from build123d import *

# Parameters (mm, degrees)
SKETCH012_W             = 34.7
SKETCH012_H             = 9.5
PAD002_DEPTH            = 10.2
SKETCH013_W             = 34.7
SKETCH013_H             = 8
POCKET010_DEPTH         = 8.4
SKETCH014_W             = 11.3
SKETCH014_H             = 8
PAD003_DEPTH            = 3.8
SKETCH015_R             = 1.5
PAD004_DEPTH            = 7.5
FILLET002_R             = 0.5
SKETCH016_W             = 8.8
SKETCH016_H             = 6.75
POCKET011_DEPTH         = 3.81
SKETCH018_W             = 1.25
SKETCH018_H             = 4
POCKET012_DEPTH         = 1.25
PAD005_DEPTH            = 2.56
SKETCH019_R             = 1.9
PAD006_DEPTH            = 5
SKETCH020_R             = 1.05
POCKET014_DEPTH         = 2.56
SKETCH021_R             = 0.75
POCKET015_DEPTH         = 5
SKETCH022_W             = 1
SKETCH022_H             = 9.5
POCKET016_DEPTH         = 0.3
SKETCH023_W             = 1
SKETCH023_H             = 10.2
POCKET017_DEPTH         = 0.3
FILLET003_R             = 0.2
FILLET004_R             = 0.2
SKETCH036_R             = 1.625
PAD012_DEPTH            = 4
FILLET008_R             = 0.5
FILLET020_R             = 0.5
PAD161_DEPTH            = 1
BODY002_ROLL_ANGLE      = -90
BODY002_PLACEMENT_ANGLE = -90


with BuildPart() as part:
    # Sketch012 → Pad002 (new body)
    with BuildSketch(Plane.XY):
        with Locations((-17.35, 0)):
            Rectangle(SKETCH012_W, SKETCH012_H)
    extrude(amount=PAD002_DEPTH)

    # Sketch013 (on Face6 of Pad002) → Pocket010 (cut)
    with BuildSketch(Plane.XY.offset(10.2)):
        with Locations((-17.35, 0.75)):
            Rectangle(SKETCH013_W, SKETCH013_H)
    extrude(amount=-POCKET010_DEPTH, mode=Mode.SUBTRACT)

    # Sketch014 (on Face6 of Pocket010) → Pad003 (join)
    with BuildSketch(Plane.XY.offset(1.8)):
        with Locations((-12.75, 0.75)):
            Rectangle(SKETCH014_W, SKETCH014_H)
    extrude(amount=PAD003_DEPTH)

    # Sketch015 (on Face6 of Pad003) → Pad004 (join)
    with BuildSketch(Plane.XY.offset(1.8)):
        with Locations((-22, 0.75)):
            Circle(SKETCH015_R)
    extrude(amount=PAD004_DEPTH)

    # Fillet002
    fillet002_edges = [part.edges().sort_by_distance(p)[0] for p in [
        (-17.35, -4.75, 0),
        (-34.7, -4.75, 5.1),
        (-34.7, 0, 0),
        (0, -4.75, 5.1),
        (0, 0, 0),
    ]]
    fillet(fillet002_edges, radius=FILLET002_R)

    # Sketch016 (on Face14 of Fillet002) → Pocket011 (cut)
    with BuildSketch(Plane.XY.offset(5.6)):
        with Locations((-12.75, 0.125)):
            Rectangle(SKETCH016_W, SKETCH016_H)
    extrude(amount=-POCKET011_DEPTH, mode=Mode.SUBTRACT)

    # Sketch018 (on Face13 of Pocket011) → Pocket012 (cut)
    with BuildSketch(Plane.XY.offset(5.6)):
        with Locations((-7.725, 0.75)):
            Rectangle(SKETCH018_W, SKETCH018_H)
    extrude(amount=-POCKET012_DEPTH, mode=Mode.SUBTRACT)

    # Sketch017 (on Face23 of Pocket011) → Pad005 (join)
    with BuildSketch(Plane.XY.offset(1.79)):
        with BuildLine():
            Line((-8.35, 2.75), (-11.5, 2.75))
            ThreePointArc((-11.5, 2.75), (-13.500002, 0.750015), (-11.500029, -1.25))
            Line((-11.500029, -1.25), (-8.35, -1.25))
            Line((-8.35, -1.25), (-8.35, 2.75))
        make_face()
    extrude(amount=PAD005_DEPTH)

    # Sketch019 (on Face16 of Pad005) → Pad006 (join)
    with BuildSketch(Plane.XY.offset(1.79)):
        with Locations((-15.5, 0.75)):
            Circle(SKETCH019_R)
    extrude(amount=PAD006_DEPTH)

    # Sketch020 (on Face26 of Pad006) → Pocket014 (cut)
    with BuildSketch(Plane.XY.offset(4.35)):
        with Locations((-11.5, 0.75)):
            Circle(SKETCH020_R)
    extrude(amount=-POCKET014_DEPTH, mode=Mode.SUBTRACT)

    # Sketch021 (on Face37 of Pocket014) → Pocket015 (cut)
    with BuildSketch(Plane.XY.offset(6.79)):
        with Locations((-15.5, 0.75)):
            Circle(SKETCH021_R)
    extrude(amount=-POCKET015_DEPTH, mode=Mode.SUBTRACT)

    # Sketch022 (on Face20 of Pocket015) → Pocket016 (cut)
    with BuildSketch(Plane(origin=(0, 0, 0), x_dir=(1, 0, 0), z_dir=(0, 0, -1))):
        with BuildLine():
            ThreePointArc((-27.95, 2.25), (-30.2, 0), (-27.95, -2.25))
            Line((-27.95, -2.25), (-11.95, -2.25))
            ThreePointArc((-11.95, -2.25), (-9.7, 0), (-11.95, 2.25))
            Line((-27.95, 2.25), (-11.95, 2.25))
        make_face()
        with Locations((-6.95, 0)):
            Rectangle(SKETCH022_W, SKETCH022_H)
    extrude(amount=-POCKET016_DEPTH, mode=Mode.SUBTRACT)

    # Sketch023 (on Face10 of Pocket016) → Pocket017 (cut)
    with BuildSketch(Plane.XZ.offset(4.75)):
        with Locations((-6.95, 5.1)):
            Rectangle(SKETCH023_W, SKETCH023_H)
    extrude(amount=-POCKET017_DEPTH, mode=Mode.SUBTRACT)

    # Fillet003
    fillet003_edges = [part.edges().sort_by_distance(p)[0] for p in [
        (-9.7, 0, 0),
        (-19.95, 2.25, 0),
        (-19.95, -2.25, 0),
        (-30.2, 0, 0),
    ]]
    fillet(fillet003_edges, radius=FILLET003_R)

    # Fillet004
    fillet004_edges = [part.edges().sort_by_distance(p)[0] for p in [
        (-7.45, 0.25, 0),
        (-6.45, 0.25, 0),
        (-7.45, -4.352155, 0.010547),
        (-7.45, -4.603553, 0.146447),
        (-7.45, -4.739453, 0.397845),
        (-7.45, -4.75, 5.35),
        (-6.45, -4.75, 5.35),
        (-6.45, -4.739453, 0.397845),
        (-6.45, -4.603553, 0.146447),
        (-6.45, -4.352155, 0.010547),
    ]]
    fillet(fillet004_edges, radius=FILLET004_R)

    # Sketch036 (on Face13 of Fillet004) → Pad012 (join)
    with BuildSketch(Plane.XZ.offset(4.75)):
        with Locations((-16.6, 5.1)):
            Circle(SKETCH036_R)
    extrude(amount=PAD012_DEPTH)

    # Fillet008
    fillet008_edges = [part.edges().sort_by_distance(p)[0] for p in [
        (-18.225, -8.75, 5.1),
    ]]
    fillet(fillet008_edges, radius=FILLET008_R)

    # Fillet020
    fillet020_edges = [part.edges().sort_by_distance(p)[0] for p in [
        (-7.1, 4.75, 3.7),
        (-18.4, 4.75, 3.7),
    ]]
    fillet(fillet020_edges, radius=FILLET020_R)

    # Sketch282 (on Face29 of Fillet020) → Pad161 (join)
    with BuildSketch(Plane.XY.offset(10.2)):
        with BuildLine():
            Line((0, -3.25), (0, -4.25))
            ThreePointArc((-0.5, -4.75), (-0.146447, -4.603553), (0, -4.25))
            Line((-0.5, -4.75), (-6.25, -4.75))
            ThreePointArc((-6.45, -4.55), (-6.391421, -4.691421), (-6.25, -4.75))
            Line((-6.45, -4.55), (-6.45, -4.45))
            Line((-6.45, -4.45), (-7.45, -4.45))
            Line((-7.45, -4.45), (-7.45, -4.55))
            ThreePointArc((-7.65, -4.75), (-7.508579, -4.691421), (-7.45, -4.55))
            Line((-7.65, -4.75), (-34.2, -4.75))
            ThreePointArc((-34.7, -4.25), (-34.553553, -4.603553), (-34.2, -4.75))
            Line((-34.7, -4.25), (-34.7, -3.25))
            Line((-34.7, -3.25), (0, -3.25))
        make_face()
    extrude(amount=PAD161_DEPTH)


with BuildPart() as part_1:
    # Body002 roll: moved
    add(part.part.rotate(Axis((0, 0, 0), (1, 0, 0)), BODY002_ROLL_ANGLE))


with BuildPart() as part_2:
    # Body002 placement: moved
    add(part_1.part.moved(Location((26.75, -55.7, 8))).rotate(Axis((26.75, -55.7, 8), (0, 0, 1)), BODY002_PLACEMENT_ANGLE))


solid = part_2.part
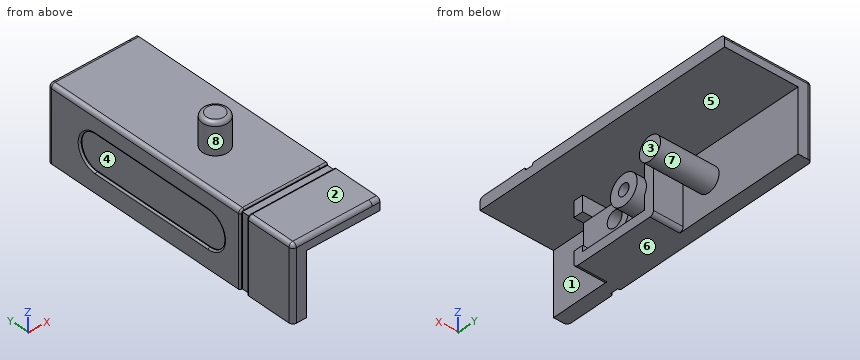
Design review of the part built by this model. Coordinates are the model's own, in mm. Face numbers are marked on the shaded views. A direction names the side the tool comes from. Coordinates: 2 decimals unless noted, no trailing zeros. Loops run counter-clockwise (first coordinate to the right, second up) from the corner with the lowest first, then second, coordinate; pieces in that order, holes last.
Item 1: Add section A-A (x = 29.5). Give the number of separate pieces and of enclosed holes in the cut face, and give its area (3 significant figures).
Completed:
separate pieces: 2
enclosed holes: 3
area: 114 mm2
Item 2: Add section C-C (x = 28). Write out the cut boundary in (y, z), and give its area (3 significant figures).
Completed:
outline: (-55.7, 3.25) - (-21, 3.25) - (-21, 12.25) arc R0.5 ccw to (-21.5, 12.75) - (-48.05, 12.75) arc R0.2 ccw to (-48.25, 12.55) - (-48.25, 12.45) - (-49.25, 12.45) - (-49.25, 12.55) arc R0.2 ccw to (-49.45, 12.75) - (-55.2, 12.75) arc R0.5 ccw to (-55.7, 12.25) - close
area: 329 mm2
Item 3: Add section B-B (y = -33.7). Write out the cut boundary in (x, z), and give its area (3 significant figures).
Completed:
outline: (26.75, 3.25) - (28.55, 3.25) - (28.55, 5.75) - (36.05, 5.75) - (36.05, 8.75) - (28.55, 8.75) - (28.55, 11.25) - (37.95, 11.25) - (37.95, 12.75) - (27.25, 12.75) arc R0.5 ccw to (26.75, 12.25) - (26.75, 10.45) arc R0.2 ccw to (26.95, 10.25) - (27.05, 10.25) - (27.05, 5.75) - (26.95, 5.75) arc R0.2 ccw to (26.75, 5.55) - close
area: 52.3 mm2
Item 4: Wall thickness on L1, parallel to Z at x = 29.8, y = -44.2; L2, parallel to Y at x = 31.2, z = 7.25; L3, parallel to Z at x = 30, y = -40.2: over which ranges is each line inside the solid? List them lowest first.
Completed:
L1: z = 3.25 to 4.5, 5.25 to 6.2, 8.3 to 9.25, 11.25 to 12.75
L2: y = -42.1 to -40.95, -39.45 to -37.3, -35.2 to -32.2
L3: z = 3.25 to 4.5, 5.35 to 6.5, 8 to 9.15, 11.25 to 12.75
Item 5: Clearance check with flat-ended pins moving along their axes: pin 1 (1.7 mm diameter, centred on y = -44, z = 7.5, fed in from +X); pin 2 (3 mm diameter, centred on x = 30.5, y = -43, fed in from +Z); pin 3 (1 mm diameter, centred on x = 35, y = -47, fed in from -Z); pin 4 (6 mm diameter, centred on x = 36.5, z = 11, fed in from +Y). State where each tip first meets the part, or that it passes through.
Completed:
pin 1: stops at x = 31.1
pin 2: stops at z = 12.75
pin 3: stops at z = 11.25
pin 4: stops at y = -21
Item 6: Draft analysis for pull direction Z (two halves, no side actions). For the marked faces 5, 6, 7 and 8, state which applies: pulls with the +Z half, pulls with the -Z half, needs draft (parallel to the pull), parting line crosses it, or undercut.
Completed:
face 5: undercut
face 6: pulls with the -Z half
face 7: undercut
face 8: needs draft
Item 7: Add section D-D (z = 15.75). Write out the cut boundary in (x, y) (3 decimals).
Completed:
outline: circle Ø3.25 at (31.85, -39.1)
Item 8: For the marked faces 1, 2, 3 and 4, list the 3-axis set-ups (+Z, -Z, +X, -X, +Y, -Y) from which the entire face can be reached by the end or side of a thin tool; tool diameter is ignored.
Completed:
face 1: -Z, +X, -Y
face 2: +Z, +X, -X, -Y
face 3: -Z, +X, +Y, -Y
face 4: -X
